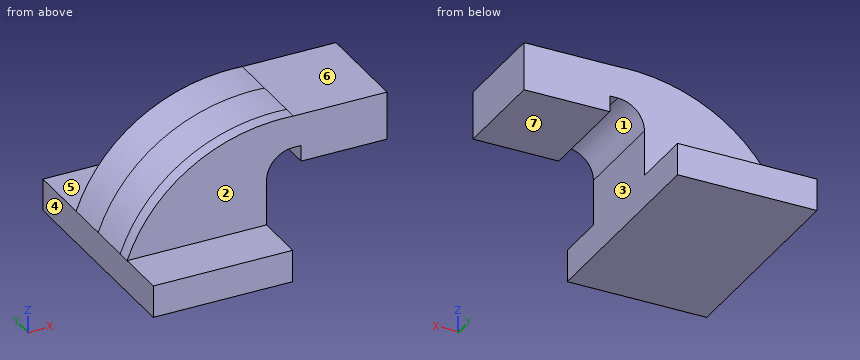
from build123d import *

# Parameters (mm, degrees)
F1_DEPTH = 63.5
F0_W     = 25.4
F0_H     = 28.575
F2_DEPTH = 25.4
F3_DEPTH = 7.9375


with BuildPart() as f1:
    # F0 (on Front) → F1 (new body, symmetric)
    with BuildSketch(Plane.XZ):
        Polygon((-41.275, 9.525), (-41.275, -9.525), (41.275, -9.525), (41.275, 9.525), (22.225, 9.525), align=None)
    extrude(amount=F1_DEPTH, both=True)

    # F0 (on Front) → F2 (join, symmetric)
    with BuildSketch(Plane.XZ):
        Polygon((-41.275, 9.525), (-41.275, -9.525), (41.275, -9.525), (41.275, 9.525), (22.225, 9.525), align=None)
        with BuildLine():
            add(Edge.make_bspline(
                [(-41.275, 9.525), (-25.692793, 51.531576), (14.306218, 73.720813), (57.15, 71.4502)],
                knots=[0, 0, 0, 0, 116.285042, 116.285042, 116.285042, 116.285042], degree=3))
            Line((-41.275, 9.525), (22.225, 9.525))
            Line((22.225, 9.525), (22.225, 36.5252))
            ThreePointArc((22.225, 36.5252), (32.454296, 61.220904), (57.15, 71.4502))
        make_face()
        with BuildLine():
            Line((22.225, 9.525), (41.275, 9.525))
            Line((41.275, 9.525), (41.275, 36.5252))
            ThreePointArc((41.275, 36.5252), (45.92468, 47.75052), (57.15, 52.4002))
            Line((57.15, 52.4002), (61.7728, 52.4002))
            Line((61.7728, 52.4002), (61.7728, 71.4502))
            Line((61.7728, 71.4502), (57.15, 71.4502))
            ThreePointArc((57.15, 71.4502), (32.454296, 61.220904), (22.225, 36.5252))
            Line((22.225, 36.5252), (22.225, 9.525))
        make_face()
        Polygon((85.725, 71.4502), (61.7728, 71.4502), (61.7728, 52.4002), (61.7728, 42.8752), (87.1728, 42.8752), (87.1728, 71.4502), align=None)
        with Locations((99.8728, 57.1627)):
            Rectangle(F0_W, F0_H)
    extrude(amount=F2_DEPTH, both=True)

    # F0 (on Front) + F2_face (on face) → F3 (join, symmetric)
    with BuildSketch(Plane.XZ):
        Polygon((-41.275, 9.525), (-41.275, -9.525), (41.275, -9.525), (41.275, 9.525), (22.225, 9.525), align=None)
        with BuildLine():
            add(Edge.make_bspline(
                [(-41.275, 9.525), (-25.692793, 51.531576), (14.306218, 73.720813), (57.15, 71.4502)],
                knots=[0, 0, 0, 0, 116.285042, 116.285042, 116.285042, 116.285042], degree=3))
            Line((-41.275, 9.525), (22.225, 9.525))
            Line((22.225, 9.525), (22.225, 36.5252))
            ThreePointArc((22.225, 36.5252), (32.454296, 61.220904), (57.15, 71.4502))
        make_face()
        with BuildLine():
            Line((22.225, 9.525), (41.275, 9.525))
            Line((41.275, 9.525), (41.275, 36.5252))
            ThreePointArc((41.275, 36.5252), (45.92468, 47.75052), (57.15, 52.4002))
            Line((57.15, 52.4002), (61.7728, 52.4002))
            Line((61.7728, 52.4002), (61.7728, 71.4502))
            Line((61.7728, 71.4502), (57.15, 71.4502))
            ThreePointArc((57.15, 71.4502), (32.454296, 61.220904), (22.225, 36.5252))
            Line((22.225, 36.5252), (22.225, 9.525))
        make_face()
        Polygon((85.725, 71.4502), (61.7728, 71.4502), (61.7728, 52.4002), (61.7728, 42.8752), (87.1728, 42.8752), (87.1728, 71.4502), align=None)
        with Locations((99.8728, 57.1627)):
            Rectangle(F0_W, F0_H)
    with BuildSketch(Plane(origin=(32.737108, -25.4, 42.563557), x_dir=(1, 0, 0), z_dir=(0, -1, 0))):
        with BuildLine():
            add(Edge.make_bspline(
                [(-74.012108, -33.038557), (-58.429901, 8.968018), (-18.43089, 31.157256), (24.412892, 28.886643)],
                knots=[0, 0, 0, 0, 116.285042, 116.285042, 116.285042, 116.285042], degree=3))
            Line((-74.012108, -33.038557), (8.537892, -33.038557))
            Line((8.537892, -33.038557), (8.537892, -6.038357))
            ThreePointArc((8.537892, -6.038357), (13.187572, 5.186963), (24.412892, 9.836643))
            Line((24.412892, 9.836643), (29.035692, 9.836643))
            Line((29.035692, 9.836643), (29.035692, 0.311643))
            Line((29.035692, 0.311643), (79.835692, 0.311643))
            Line((79.835692, 0.311643), (79.835692, 28.886643))
            Line((79.835692, 28.886643), (24.412892, 28.886643))
        make_face()
    extrude(amount=F3_DEPTH, both=True)


solid = f1.part
Part model, mm, in its own coordinate system. Face numbers are marked on the shaded views. A direction names the side the tool comes from. Give positions to 0.01 mm unless a question says otherwise; leave off trailing zeros. Order: outer loops, then holes, each group sorted by start corner. A loop starts at its lowest first (then second) coordinate and runs counter-clockwise, first axis right, second up. Notation, with made-up numbers: (59.25, 53) - (86.25, 53) arc R26 ccw to (86.25, 91) - close; hole circle Ø8 at (4, 3). An arc over 180 degrees is marked (long way). Use a Markdown table: item, result.
1) Saw through at B-B on x = 97.5. List the corners of the cut face in (y, z).
Checked values:
| item | result |
|---|---|
| outline | (-33.34, 42.88) - (25.4, 42.88) - (25.4, 71.45) - (-33.34, 71.45) - close |
2) Flat gauge pins, fed straight in: P1, Ø2, axis at y = 17, z = 21, coming from the +X side (3 decimals); P2, Ø5, axis at x = 10, z = 34.5, coming from the +Y side; P3, Ø1.4, axis at x = 60, y = 3, coming from the -Z side. Where does each tip first touch, or does it go through?
Checked values:
| item | result |
|---|---|
| P1 | x = 41.275 |
| P2 | y = 25.4 |
| P3 | z = 52.4 |
3) Probe L1, parallel to Z at x = 26.5, y = -56.5 (3 decimals); L2, parallel to Y at x = 32.5, z = 39; L3, parallel to Z at x = 90.5, y = -6.5. List the from-to ranges inside material, lowest first. Write a range as from..to.
Checked values:
| item | result |
|---|---|
| L1 | -9.525..9.525 |
| L2 | -33.34..25.4 |
| L3 | 42.88..71.45 |
4) Two-plate mould, pull along X, no slides. Class the marked faces 1, 2, 3 and 4: +X half, -X half, draft (parallel to the pull), parting line (faces both ways), or undercut.
Checked values:
| item | result |
|---|---|
| face 1 | undercut |
| face 2 | draft |
| face 3 | +X half |
| face 4 | -X half |
5) 3-axis set-ups, long thin cutter, end or side, ignore diameter. For the marked faces 5, 6 and 7: which of +Z, -Z, +X, -X, +Y, -Y reach the whole face in a straight line?
Checked values:
| item | result |
|---|---|
| face 5 | +Z, +X, -X, +Y |
| face 6 | +Z, +X, +Y, -Y |
| face 7 | -Z, +X, +Y, -Y |
6) Saw through at A-A on z = -3. List the corners of the cut face in (x, y) (3 decimals).
Checked values:
| item | result |
|---|---|
| outline | (-41.275, -63.5) - (41.275, -63.5) - (41.275, 63.5) - (-41.275, 63.5) - close |
